CAD build for the part. Positions are in the model's coordinates, mm. Round coordinates to 2 decimals unless told otherwise and drop trailing zeros. Write each loop counter-clockwise with the first axis right and the second up, starting at its lowest first coordinate (ties: lowest second). Pieces come first, ordered by that corner, then holes. Notation, with made-up numbers: (57, 29.25) -> (71, 29.25) arc R20 cw to (71, 53.25) -> close; hole circle Ø5 at (-10.5, -17.75). An arc over 180 degrees is marked (long way). Put each result on its own line as item: value. Start each with the question number.
1. Saw through at B-B on x = -2.5. List the corners of the cut face in (y, z).
2. Drill centre lines: line 1 (Z direction, x = 12.5, y = -1.05); line 2 (X direction, y = -2.05, z = 26); line 3 (Z direction, x = 24.5, y = -2.45). Where is each one in solid material? Low to high. Write a range as from..to.
3. Saw through at D-D on y = -0.85. List the corners of the cut face in (x, z).
4. Flat gauge pin, fed straight in: P1, Ø4.5, axis at x = 12.5, z = 10, coming from the +Y side. Where does the tip first touch, or does it go through?
5. Saw through at A-A on z = 85.5. List the corners of the cut face in (x, y).
6. Saw through at C-C on x = 12.5. List the corners of the cut face in (y, z), and give its area (3 significant figures).
from build123d import *

# Parameters (mm, degrees)
F0_R     = 2.55
F0_W     = 26
F0_H     = 15
F0_R_2   = 4
F1_DEPTH = 4


with BuildPart() as f1:
    # F0 (on Front) → F1 (new body)
    with BuildSketch(Plane.XZ):
        with BuildLine():
            Line((-17.5, 93), (-17.5, 5))
            ThreePointArc((-17.5, 5), (-16.035534, 1.464466), (-12.5, 0))
            Line((-12.5, 0), (25.5, 0))
            ThreePointArc((25.5, 0), (29.035534, 1.464466), (30.5, 5))
            Line((30.5, 5), (30.5, 93))
            ThreePointArc((30.5, 93), (29.035534, 96.535534), (25.5, 98))
            Line((25.5, 98), (-12.5, 98))
            ThreePointArc((-12.5, 98), (-16.035534, 96.535534), (-17.5, 93))
        make_face()
        with Locations((12.5, 10)):
            Circle(F0_R, mode=Mode.SUBTRACT)
        with Locations((12.5, 23.05)):
            Rectangle(F0_W, F0_H, mode=Mode.SUBTRACT)
        with Locations((-2.5, 65.5)):
            Circle(F0_R_2, mode=Mode.SUBTRACT)
        with Locations((12.5, 85.5)):
            Circle(F0_R_2, mode=Mode.SUBTRACT)
    extrude(amount=F1_DEPTH)


solid = f1.part
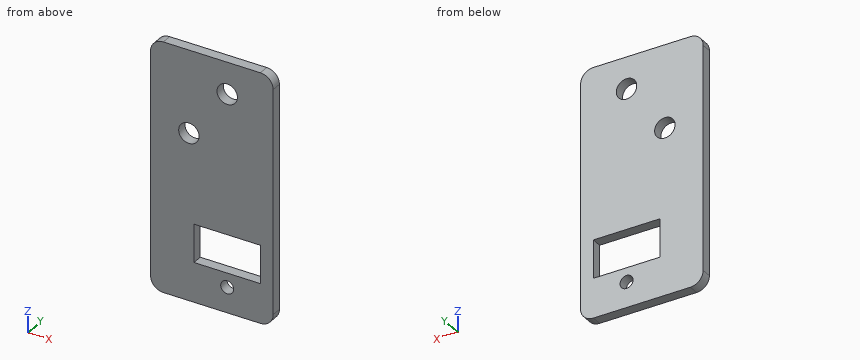
Return value:
1. outline: (-4, 0) -> (0, 0) -> (0, 61.5) -> (-4, 61.5) -> close; (-4, 69.5) -> (0, 69.5) -> (0, 98) -> (-4, 98) -> close
2. line 1: z = 0..7.45, 12.55..15.55, 30.55..81.5, 89.5..98
2. line 2: x = -17.5..-0.5, 25.5..30.5
2. line 3: z = 0..15.55, 30.55..98
3. outline: (-17.5, 5) arc R5 ccw to (-12.5, 0) -> (25.5, 0) arc R5 ccw to (30.5, 5) -> (30.5, 93) arc R5 ccw to (25.5, 98) -> (-12.5, 98) arc R5 ccw to (-17.5, 93) -> close; hole circle Ø8 at (-2.5, 65.5); hole (-0.5, 15.55) -> (25.5, 15.55) -> (25.5, 30.55) -> (-0.5, 30.55) -> close; hole circle Ø8 at (12.5, 85.5); hole circle Ø5.1 at (12.5, 10)
4. P1: passes through
5. outline: (-17.5, -4) -> (8.5, -4) -> (8.5, 0) -> (-17.5, 0) -> close; (16.5, -4) -> (30.5, -4) -> (30.5, 0) -> (16.5, 0) -> close
6. outline: (-4, 0) -> (0, 0) -> (0, 7.45) -> (-4, 7.45) -> close; (-4, 12.55) -> (0, 12.55) -> (0, 15.55) -> (-4, 15.55) -> close; (-4, 30.55) -> (0, 30.55) -> (0, 81.5) -> (-4, 81.5) -> close; (-4, 89.5) -> (0, 89.5) -> (0, 98) -> (-4, 98) -> close
6. area: 280 mm^2
